Input: dimensioned drawing with shaded views. Units: mm. Origin: part minimum x, y, z. A direction names the side the tool comes from. Round coordinates to 2 decimals unless told otherwise and drop trailing zeros. Loops run counter-clockwise (first coordinate to the right, second up) from the corner with the lowest first, then second, coordinate; pieces in that order, holes last. Notation, with made-up numbers: (33.25, -1.5) - (65.25, -1.5) arc R11 ccw to (65.25, 8.5) - close; hole circle Ø8 at (63.25, 84). An arc over 180 degrees is marked (long way). Answer as a JSON object with one key per item and string values. Group by question number.
Item 1: Draft query along X for the marked faces 3, 4 and 5. Return one class per face: released by +X, released by -X, zero draft, split by the parting line, or undercut.
Item 2: Section A-A (y = 2). Return the cut outline in (x, z).
Item 3: Reachability of the marked faces 1 and 2 from +Z, -Z, +X, -X, +Y, -Y: full face, straight path, thin tool, end or side. Return the list, or none.
Item 4: First-contact query: pin 1 (1.5 mm diameter, centred on y = 0.5, z = 1.5, fed in from +X). Flat tip, straight axial feed; report the tip coordinate or a pass-through.
Item 5: Section D-D (z = 10.75). Return the cut outline in (x, y), plus the area to 3 significant figures.
Item 6: Line query: line 1 (Y direction, x = 2, z = 3.05); line 2 (Z direction, x = 1.55, y = 2.2); line 3 (Z direction, x = 3.3, y = 2.2). Output: solid intervals per line, ascending.
Item 7: Section C-C (z = 8). Return the cut outline in (x, y).
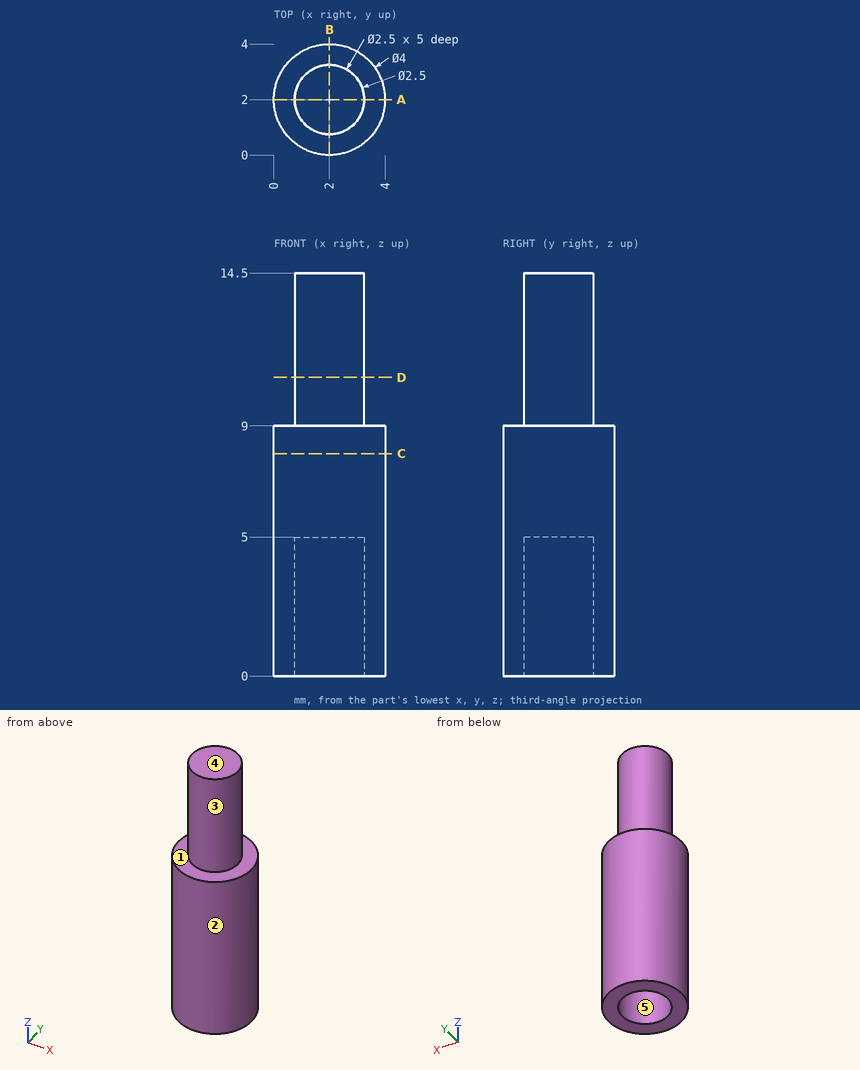
Values:
{
 "1": {"face 3": "split by the parting line", "face 4": "zero draft", "face 5": "undercut"},
 "2": {"outline": "(0, 0) - (0.75, 0) - (0.75, 5) - (3.25, 5) - (3.25, 0) - (4, 0) - (4, 9) - (3.25, 9) - (3.25, 14.5) - (0.75, 14.5) - (0.75, 9) - (0, 9) - close"},
 "3": {"face 1": "+Z", "face 2": "+Z, -Z"},
 "4": {"pin 1": "stops at x = 3.85"},
 "5": {"outline": "circle Ø2.5 at (2, 2)", "area": "4.91 mm^2"},
 "6": {"line 1": "y = 0 to 0.75, 3.25 to 4", "line 2": "z = 5 to 14.5", "line 3": "z = 0 to 9"},
 "7": {"outline": "circle Ø4 at (2, 2)"}
}
